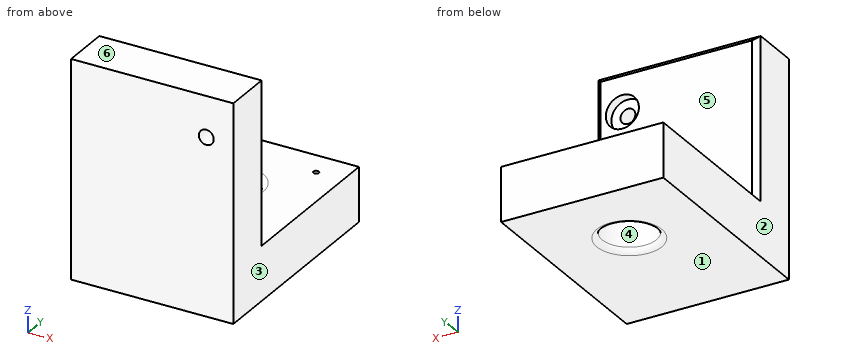
from build123d import *

# Parameters (mm, degrees)
SKETCH1_W           = 60
SKETCH1_H           = 60
BOSS_EXTRUDE1_DEPTH = 20
SKETCH1_3_W         = 60
SKETCH1_3_H         = 20
BOSS_EXTRUDE2_DEPTH = 80
SKETCH3_R           = 10
CUT_EXTRUDE2_DEPTH  = 117.619037897
FILLET2_R           = 2
SKETCH4_R           = 1
CUT_EXTRUDE3_DEPTH  = 10
SKETCH7_R           = 6.12
CUT_EXTRUDE5_DEPTH  = 3.58
SKETCH8_R           = 2.75
CUT_EXTRUDE6_DEPTH  = 107.030261718
CUT_EXTRUDE7_DEPTH  = 60
FILLET7_R           = 2
CUT_EXTRUDE13_DEPTH = 60


with BuildPart() as part:
    # Sketch1 → Boss-Extrude1 (new body)
    with BuildSketch(Plane(origin=(0, 0, 0), x_dir=(1, 0, 0), z_dir=(0, 1, 0))):
        with Locations((30, -30)):
            Rectangle(SKETCH1_W, SKETCH1_H)
    extrude(amount=BOSS_EXTRUDE1_DEPTH)

    # Sketch1_3 → Boss-Extrude2 (add)
    with BuildSketch(Plane(origin=(0, 0, 0), x_dir=(1, 0, 0), z_dir=(0, 1, 0))):
        with Locations((30, 10)):
            Rectangle(SKETCH1_3_W, SKETCH1_3_H)
    extrude(amount=BOSS_EXTRUDE2_DEPTH)

    # Sketch3 → Cut-Extrude2 (cut, through all)
    with BuildSketch(Plane.XY):
        with Locations((30, 50)):
            Circle(SKETCH3_R)
    extrude(amount=-CUT_EXTRUDE2_DEPTH, mode=Mode.SUBTRACT)

    # Fillet2
    fillet2_edges = [part.edges().sort_by_distance(p)[0] for p in [
        (20, 50, -20),
        (20, 50, 0),
    ]]
    fillet(fillet2_edges, radius=FILLET2_R)

    # Sketch4 → Cut-Extrude3 (cut)
    with BuildSketch(Plane.XY):
        with Locations((10, 70)):
            Circle(SKETCH4_R)
        with Locations((50, 70)):
            Circle(SKETCH4_R)
        with Locations((50, 30)):
            Circle(SKETCH4_R)
        with Locations((10, 30)):
            Circle(SKETCH4_R)
    extrude(amount=-CUT_EXTRUDE3_DEPTH, mode=Mode.SUBTRACT)

    # Sketch7 → Cut-Extrude5 (cut)
    with BuildSketch(Plane(origin=(0, 20, 0), x_dir=(1, 0, 0), z_dir=(0, 1, 0))):
        with Locations(Location((50, -45, 0), (0, 0, 270))):
            Circle(SKETCH7_R)
    extrude(amount=-CUT_EXTRUDE5_DEPTH, mode=Mode.SUBTRACT)

    # Sketch8 → Cut-Extrude6 (cut, through all)
    with BuildSketch(Plane(origin=(0, 16.42, 0), x_dir=(1, 0, 0), z_dir=(0, 1, 0))):
        with Locations(Location((50, -45, 0), (0, 0, 270))):
            Circle(SKETCH8_R)
    extrude(amount=-CUT_EXTRUDE6_DEPTH, mode=Mode.SUBTRACT)

    # Sketch9 → Cut-Extrude7 (cut)
    with BuildSketch(Plane.XY.offset(60)):
        Polygon((0, 20), (2, 20), (0, 18), align=None)
        Polygon((60, 20), (58, 20), (60, 18), align=None)
    extrude(amount=-CUT_EXTRUDE7_DEPTH, mode=Mode.SUBTRACT)

    # Fillet7
    fillet7_edges = [part.edges().sort_by_distance(p)[0] for p in [
        (30, 20, 0),
    ]]
    fillet(fillet7_edges, radius=FILLET7_R)

    # Sketch11 → Cut-Extrude13 (cut)
    with BuildSketch(Plane(origin=(60, 0, 0), x_dir=(0, 0, -1), z_dir=(1, 0, 0))):
        Polygon((-60, 20), (-58, 20), (-60, 18), align=None)
    extrude(amount=-CUT_EXTRUDE13_DEPTH, mode=Mode.SUBTRACT)


solid = part.part
Model file for the job. Use its own axes, mm. Face numbers are marked on the shaded views. A direction names the side the tool comes from. Give positions to 0.01 mm unless a question says otherwise; leave off trailing zeros. Loops run counter-clockwise (first coordinate to the right, second up) from the corner with the lowest first, then second, coordinate; pieces in that order, holes last. Notation, with made-up numbers: (36.5, 43.25) -> (63.5, 43.25) arc R23 ccw to (63.5, 56.25) -> close; hole circle Ø8 at (27, 81.25). An arc over 180 degrees is marked (long way). Use a Markdown table: item, result. Add a question column.
(1) Slice it at A-A on z = 45. List the corners of the cut face in (x, y), and give its area (3 significant figures).
(2) Tool access for the marked faces 5 and 6: list every direction of +Z, -Z, +X, -X, +Y, -Y with a clear straight run to the whole face (end or side of a thin tool).
(3) Mould opens along X. For the marked faces 1, 2, 3 and 4 say: +X half, -X half, draft (parallel to the pull), parting line (faces both ways), or undercut.
(4) Slice it at B-B on z = -6.5. List the corners of the cut face in (x, y).
(5) Drop flat-ended pins along their axis: pin 1 Ø2.5 at (x, y) = (50, 30) entering from +Z; pin 2 Ø23 at (x, y) = (30, 50) entering from -Z; pin 3 Ø0.6 at (x, y) = (50.5, 30) entering from +Z. Give the stop position or say it passes through.
(6) Wall check: line 1 along Y through (x, z) = (50, -4.5); line 2 along X through (y, z) = (70, -7); line 3 along Y through (x, z) = (30, -12). Give the ranges that are in metal, low to high.
Filled sheet:
| question | item | result |
|---|---|---|
| 1 | outline | (0, 0) -> (47.25, 0) -> (47.25, 16.42) -> (43.88, 16.42) -> (43.88, 20) -> (2, 20) -> (0, 18) -> close; (52.75, 0) -> (60, 0) -> (60, 18) -> (58, 20) -> (56.12, 20) -> (56.12, 16.42) -> (52.75, 16.42) -> close |
| 1 | area | 1,060 mm2 |
| 2 | face 5 | +Z, +X, -X, +Y |
| 2 | face 6 | +Z, +X, -X, +Y, -Y |
| 3 | face 1 | draft |
| 3 | face 2 | -X half |
| 3 | face 3 | +X half |
| 3 | face 4 | undercut |
| 4 | outline | (0, 0) -> (60, 0) -> (60, 80) -> (0, 80) -> close; hole circle Ø2 at (10, 30); hole circle Ø2 at (10, 70); hole circle Ø20 at (30, 50); hole circle Ø2 at (50, 30); hole circle Ø2 at (50, 70) |
| 5 | pin 1 | z = 0 |
| 5 | pin 2 | z = -19.94 |
| 5 | pin 3 | z = -10 |
| 6 | line 1 | 0 to 29, 31 to 69, 71 to 80 |
| 6 | line 2 | 0 to 9, 11 to 49, 51 to 60 |
| 6 | line 3 | 0 to 40, 60 to 80 |
